```python
from build123d import *

# Parameters (mm, degrees)
BOSS_EXTRUDE1_DEPTH = 12.5
FILLET1_R           = 15
SKETCH2_R           = 2.1
CUT_EXTRUDE1_DEPTH  = 5
CUT_EXTRUDE2_DEPTH  = 2.5
SKETCH4_R           = 1.6
CUT_EXTRUDE3_DEPTH  = 5
CUT_EXTRUDE4_DEPTH  = 2.5
SKETCH6_R           = 1.6
CUT_EXTRUDE5_DEPTH  = 49.75282328
CUT_EXTRUDE6_DEPTH  = 2.5


with BuildPart() as part:
    # Sketch1 → Boss-Extrude1 (new body)
    with BuildSketch(Plane.XY):
        Polygon((38.266666667, 27.5), (38.266666667, 22.5), (5, 22.5), (5, -22.5), (38.266666667, -22.5), (38.266666667, -27.5), (0, -27.5), (0, 27.5), align=None)
    extrude(amount=BOSS_EXTRUDE1_DEPTH)

    # Fillet1
    fillet1_edges = [part.edges().sort_by_distance(p)[0] for p in [
        (5, 22.5, 6.25),
        (5, -22.5, 6.25),
    ]]
    fillet(fillet1_edges, radius=FILLET1_R)

    # Sketch2 → Cut-Extrude1 (cut)
    with BuildSketch(Plane(origin=(0, 27.5, 0), x_dir=(1, 0, 0), z_dir=(0, 1, 0))):
        with Locations(Location((28.266666667, -6.25, 0), (0, 0, 270))):
            Circle(SKETCH2_R)
    extrude(amount=-CUT_EXTRUDE1_DEPTH, mode=Mode.SUBTRACT)

    # Sketch3 → Cut-Extrude2 (cut)
    with BuildSketch(Plane.XZ.offset(-22.5)):
        Polygon((30.345127636, 9.85), (26.188205698, 9.85), (24.109744729, 6.25), (26.188205698, 2.65), (30.345127636, 2.65), (32.423588605, 6.25), align=None)
    extrude(amount=-CUT_EXTRUDE2_DEPTH, mode=Mode.SUBTRACT)

    # Sketch4 → Cut-Extrude3 (cut)
    with BuildSketch(Plane(origin=(0, -22.5, 0), x_dir=(1, 0, 0), z_dir=(0, 1, 0))):
        with Locations(Location((28.266666667, -6.25, 0), (0, 0, 180))):
            Circle(SKETCH4_R)
    extrude(amount=-CUT_EXTRUDE3_DEPTH, mode=Mode.SUBTRACT)

    # Sketch5 → Cut-Extrude4 (cut)
    with BuildSketch(Plane(origin=(0, -22.5, 0), x_dir=(1, 0, 0), z_dir=(0, 1, 0))):
        Polygon((29.912114934, -3.4), (26.621218399, -3.4), (24.975770132, -6.25), (26.621218399, -9.1), (29.912114934, -9.1), (31.557563201, -6.25), align=None)
    extrude(amount=-CUT_EXTRUDE4_DEPTH, mode=Mode.SUBTRACT)

    # Sketch6 → Cut-Extrude5 (cut, through all)
    with BuildSketch(Plane(origin=(38.266666667, 0, 0), x_dir=(0, 0, -1), z_dir=(1, 0, 0))):
        with Locations(Location((-6.25, 0, 0), (0, 0, 90))):
            Circle(SKETCH6_R)
    extrude(amount=-CUT_EXTRUDE5_DEPTH, mode=Mode.SUBTRACT)

    # Sketch7 → Cut-Extrude6 (cut)
    with BuildSketch(Plane(origin=(5, 0, 0), x_dir=(0, 0, -1), z_dir=(1, 0, 0))):
        Polygon((-3.4, -1.645448267), (-3.4, 1.645448267), (-6.25, 3.290896534), (-9.1, 1.645448267), (-9.1, -1.645448267), (-6.25, -3.290896534), align=None)
    extrude(amount=-CUT_EXTRUDE6_DEPTH, mode=Mode.SUBTRACT)


solid = part.part
```
Can you work these out from the model? Positions are in its coordinate system, mm. A direction names the side the tool comes from. Coordinates: 2 decimals unless noted, no trailing zeros. Write each loop counter-clockwise with the first axis right and the second up, starting at its lowest first coordinate (ties: lowest second). Pieces come first, ordered by that corner, then holes. Notation, with made-up numbers: (69, 0.25) - (107, 0.25) arc R16 cw to (107, 11.25) - close; hole circle Ø6 at (34.5, -18). An arc over 180 degrees is marked (long way). Return JSON: item names as keys, results as strings.
Q1. Please list where these lines run through material, in increasing order: L1, parallel to Z at x = 1.15, y = 0; L2, parallel to Y at x = 25.5, z = 4.25; L3, parallel to X at y = 27, z = 6.25. Write a range as from..to.
Computed values:
{"L1": "z = 0..4.65, 7.85..12.5", "L2": "y = -27.5..-22.5, 25..27.5", "L3": "x = 0..26.17, 30.37..38.27"}
Q2. If we section it at C-C (x = 8): Please give me the cut outline in (y, z).
Computed values:
{"outline": "(-27.5, 0) - (-16.5, 0) - (-16.5, 12.5) - (-27.5, 12.5) - close; (16.5, 0) - (27.5, 0) - (27.5, 12.5) - (16.5, 12.5) - close"}
Q3. Thinking about a two-plate mould opening in Y: for faces 5 (the flat face through (19, 27.5, 6)), 6 (the flat face through (4, -2, 0)), 7 (the flat face through (30.746, -23.732, 4.845)), which applies, +Y half, -Y half, draft (parallel to the pull), parting line (faces both ways), or undercut?
Computed values:
{"face 5": "+Y half", "face 6": "draft", "face 7": "undercut"}
Q4. I'm going to push flat-ended pins straight in: pin 1 Ø6.5 at (y, z) = (-1, 6) entering from +X; pin 2 Ø2.5 at (x, z) = (28.27, 6.25) entering from -Y; pin 3 Ø6 at (x, z) = (27, 7) entering from +Y; pin 4 Ø5 at (y, z) = (0, 6.25) entering from +X. Where does each tip first touch, or does it pass through?
Computed values:
{"pin 1": "stops at x = 5", "pin 2": "passes through", "pin 3": "stops at y = 27.5", "pin 4": "stops at x = 2.5"}
Q5. If we section it at D-D (z = 7): Count the separate pieces of the cut face and the enclosed holes in it, then the cut area to 3 significant figures.
Computed values:
{"separate pieces": "4", "enclosed holes": "0", "area": "633 mm2"}
Q6. On a 3-axis mill with a long thin cutter (end or side, diameter ignored), from which of +Z, -Z, +X, -X, +Y, -Y can I reach the whole of each face in a straight line? I mean faces 1 (the cylindrical face through (26.217, 26.268, 5.795)), 2 (the flat face through (2.5, 2, 7)), 3 (the cylindrical face through (9.51, 18.22, 6.34)), 4 (the flat face through (28, -24, 9.1)). Say none if no direction works.
Computed values:
{"face 1": "+Y", "face 2": "+X", "face 3": "+Z, -Z, +X", "face 4": "none"}
Q7. If we section it at A-A (x = 22.5): Please give me the cut outline in (y, z).
Computed values:
{"outline": "(-27.5, 0) - (-22.5, 0) - (-22.5, 12.5) - (-27.5, 12.5) - close; (22.5, 0) - (27.5, 0) - (27.5, 12.5) - (22.5, 12.5) - close"}
Q8. If we section it at B-B (y = 0): Please give me the cut outline in (x, z), then the cut area to 4 significant figures.
Computed values:
{"outline": "(0, 0) - (5, 0) - (5, 3.4) - (2.5, 3.4) - (2.5, 4.65) - (0, 4.65) - close; (0, 7.85) - (2.5, 7.85) - (2.5, 9.1) - (5, 9.1) - (5, 12.5) - (0, 12.5) - close", "area": "40.25 mm2"}
